Geometry check sheet. Reference: drawing and pictorial views, mm from the part's lowest x, y, z. Round coordinates to 2 decimals unless told otherwise and drop trailing zeros. Write each loop counter-clockwise with the first axis right and the second up, starting at its lowest first coordinate (ties: lowest second). Pieces come first, ordered by that corner, then holes. Notation, with made-up numbers: M 37.25,-31.75 L 57.25,-31.75 A15 ccw 57.25,-17.75 Z; hole C 9.5,78 d8. An arc over 180 degrees is marked long. Answer in a Markdown table with one row per item. Add a question column.
1. Sectioned sample at B-B on x = 110. Record the cut outline in (y, z).
2. Go/stop test with a flat-tipped pin: pin 1 Ø2 at (x, y) = (72.5, 5) entering from -Z. Record where the tip stops, or that it passes through.
3. Sectioned sample at C-C on y = 4.75. Record the cut outline in (x, z), plus the area to 3 significant figures.
4. Material ranges on probe 1 along X at (y, z) = (5.5, 40); probe 2 along Z at (x, y) = (110, 5.5); probe 3 along Z at (x, y) = (130, 5.25), recorded low to high.
5. Sectioned sample at A-A on z = 40. Record the cut outline in (x, y).
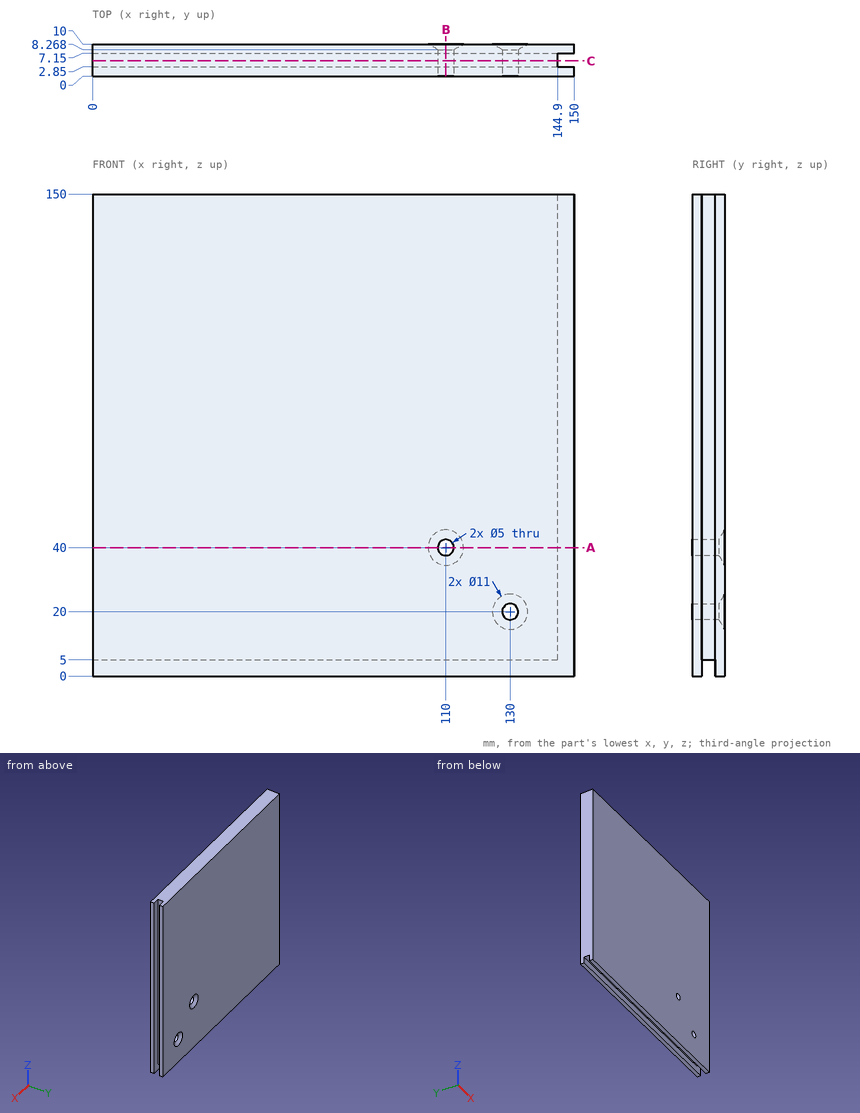
Geometry check:
| question | item | result |
|---|---|---|
| 1 | outline | M 0,0 L 2.85,0 L 2.85,5 L 7.15,5 L 7.15,0 L 10,0 L 10,34.5 L 8.27,37.5 L 0,37.5 Z; M 0,42.5 L 8.27,42.5 L 10,45.5 L 10,150 L 0,150 Z |
| 2 | pin 1 | stops at z = 5 |
| 3 | outline | M 0,5 L 144.9,5 L 144.9,150 L 0,150 Z; hole C 110,40 d5; hole C 130,20 d5 |
| 3 | area | 21,000 mm2 |
| 4 | probe 1 | x = 0 to 107.5, 112.5 to 144.9 |
| 4 | probe 2 | z = 5 to 37.5, 42.5 to 150 |
| 4 | probe 3 | z = 5 to 17.5, 22.5 to 150 |
| 5 | outline | M 0,0 L 107.5,0 L 107.5,8.27 L 104.5,10 L 0,10 Z; M 112.5,0 L 150,0 L 150,2.85 L 144.9,2.85 L 144.9,7.15 L 150,7.15 L 150,10 L 115.5,10 L 112.5,8.27 Z |
